```python
from build123d import *

# Parameters (mm, degrees)
BOSS_EXTRUDE1_DEPTH = 16.2
SKETCH2_R           = 7.5
BOSS_EXTRUDE2_DEPTH = 7
SKETCH3_R           = 4
BOSS_EXTRUDE3_DEPTH = 5
SKETCH4_R           = 2.5
CUT_EXTRUDE1_DEPTH  = 20
CHAMFER1_SIZE       = 0.6
SCALE1_SCALE        = 0.4


with BuildPart() as part:
    # Sketch1 → Boss-Extrude1 (new body)
    with BuildSketch(Plane.XY):
        Polygon((2.857883832, -4.95), (5.715767665, 0), (2.857883832, 4.95), (-2.857883832, 4.95), (-5.715767665, 0), (-2.857883832, -4.95), align=None)
    extrude(amount=BOSS_EXTRUDE1_DEPTH)

    # Sketch2 → Boss-Extrude2 (add)
    with BuildSketch(Plane.XY):
        Circle(SKETCH2_R)
    extrude(amount=-BOSS_EXTRUDE2_DEPTH)

    # Sketch3 → Boss-Extrude3 (add)
    with BuildSketch(Plane(origin=(0, 0, -7), x_dir=(-1, 0, 0), z_dir=(0, 0, -1))):
        with BuildLine():
            Line((-18, 9), (18, 9))
            ThreePointArc((18, 9), (27, 0), (18, -9))
            Line((18, -9), (-18, -9))
            ThreePointArc((-18, -9), (-27, 0), (-18, 9))
        make_face()
        with Locations((-18, 0)):
            Circle(SKETCH3_R, mode=Mode.SUBTRACT)
        with Locations((18, 0)):
            Circle(SKETCH3_R, mode=Mode.SUBTRACT)
    extrude(amount=BOSS_EXTRUDE3_DEPTH)

    # Sketch4 → Cut-Extrude1 (cut)
    with BuildSketch(Plane.XY.offset(16.2)):
        Circle(SKETCH4_R)
    extrude(amount=-CUT_EXTRUDE1_DEPTH, mode=Mode.SUBTRACT)

    # Chamfer1
    chamfer1_edges = [part.edges().sort_by_distance(p)[0] for p in [
        (4.286825749, 2.475, 16.2),
        (0, 4.95, 16.2),
        (-7.5, 0, 0),
        (-4.286825749, 2.475, 16.2),
        (-4.286825749, -2.475, 16.2),
        (27, 0, -12),
        (0, -9, -12),
        (-27, 0, -12),
        (0, 9, -12),
        (22, 0, -7),
        (-14, 0, -7),
        (27, 0, -7),
        (0, -9, -7),
        (-27, 0, -7),
        (0, 9, -7),
        (22, 0, -12),
        (-14, 0, -12),
        (-2.5, 0, 16.2),
        (0, -4.95, 16.2),
        (4.286825749, -2.475, 16.2),
    ]]
    chamfer(chamfer1_edges, length=CHAMFER1_SIZE)


with BuildPart() as part_1:
    # Scale1: scaled about (0, 0, -5.408282587)
    add(part.part.scale(SCALE1_SCALE).moved(Location((0, 0, -3.244969552))))


solid = part_1.part
```
Model file for the job. Use its own axes, mm. A direction names the side the tool comes from. Give positions to 0.01 mm unless a question says otherwise; leave off trailing zeros. Order: outer loops, then holes, each group sorted by start corner. A loop starts at its lowest first (then second) coordinate and runs counter-clockwise, first axis right, second up.
1) Wall check: probe 1 along Y at (x, z) = (-7.2, -7.25); probe 2 along Z at (x, y) = (7.5, -2.25); probe 3 along Z at (x, y) = (0, 2.25). Give the ranges that are in metal, low to high.
2) Saw through at C-C, the plane z = -1. Write the cut outline in (x, y), then the cut area to 3 significant figures.
3) 3-axis set-ups, long thin cutter, end or side, ignore diameter. For faces 5 (the cylindrical face through (0, -1, -1)), 6 (the cylindrical face through (10.8, -0.1, -7)), 7 (the flat face through (0, -1.98, 0)), 8 (the flat face through (1.71, -1, -0.17)): which of +Z, -Z, +X, -X, +Y, -Y reach the whole face in a straight line?
4) Mould opens along Y. For faces 1 (the flat face through (-1.71, 1, -0.17)), 2 (the flat face through (0, -3.6, -7)), 3 (the cylindrical face through (5.674, 0.481, -7.034)), 4 (the conical face through (10.677, -0.076, -6.163)) say: +Y half, -Y half, draft (parallel to the pull), parting line (faces both ways), or undercut.
5) Saw through at A-A, the plane z = -7.5. Write the cut outline in (x, y).
6) Saw through at B-B, the plane x = 0. Write the cut outline in (y, z).
7) Saw through at D-D, the plane y = 0.25. Count the separate pieces of the cut face and the enclosed holes in it, then the cut area to 3 significant figures.
8) Pin check, flat tips, straight feed: pin 1 (1.1 mm diameter, centred on x = 0.5, z = -1, fed in from -Y); pin 2 (1 mm diameter, centred on y = -0.5, z = -4, fed in from +X); pin 3 (1 mm diameter, centred on x = -7, y = -1.5, fed in from +Z); pin 4 (3 mm diameter, centred on x = -7.2, y = 0, fed in from -Z). Stop position of each tip, or through.
Computed:
1. probe 1: y = -3.6 to -1.6, 1.6 to 3.6
1. probe 2: z = -8.04 to -6.04
1. probe 3: z = -8.04 to -3.24
2. outline: (-2.29, 0) - (-1.14, -1.98) - (1.14, -1.98) - (2.29, 0) - (1.14, 1.98) - (-1.14, 1.98) - close; hole circle Ø2 at (0, 0)
2. area: 10.4 mm2
3. face 5: +Z
3. face 6: +Z, -Z, +X
3. face 7: +Z, +X, -X, -Y
3. face 8: +Z, +X, -Y
4. face 1: +Y half
4. face 2: -Y half
4. face 3: undercut
4. face 4: parting line
5. outline: (-7.2, -3.6) - (7.2, -3.6) arc R3.6 ccw to (7.2, 3.6) - (-7.2, 3.6) arc R3.6 ccw to start; hole circle Ø3.2 at (-7.2, 0); hole circle Ø3.2 at (7.2, 0)
6. outline: (-3.6, -7.8) - (-3.36, -8.04) - (3.36, -8.04) - (3.6, -7.8) - (3.6, -6.28) - (3.36, -6.04) - (3, -6.04) - (3, -3.48) - (2.76, -3.24) - (1.98, -3.24) - (1.98, 3) - (1.74, 3.24) - (1.24, 3.24) - (1, 3) - (1, -4.76) - (-1, -4.76) - (-1, 3) - (-1.24, 3.24) - (-1.74, 3.24) - (-1.98, 3) - (-1.98, -3.24) - (-2.76, -3.24) - (-3, -3.48) - (-3, -6.04) - (-3.36, -6.04) - (-3.6, -6.28) - close
7. separate pieces: 3
7. enclosed holes: 0
7. area: 59.0 mm2
8. pin 1: stops at y = -1.98
8. pin 2: stops at x = 3
8. pin 3: stops at z = -6.04
8. pin 4: passes through
